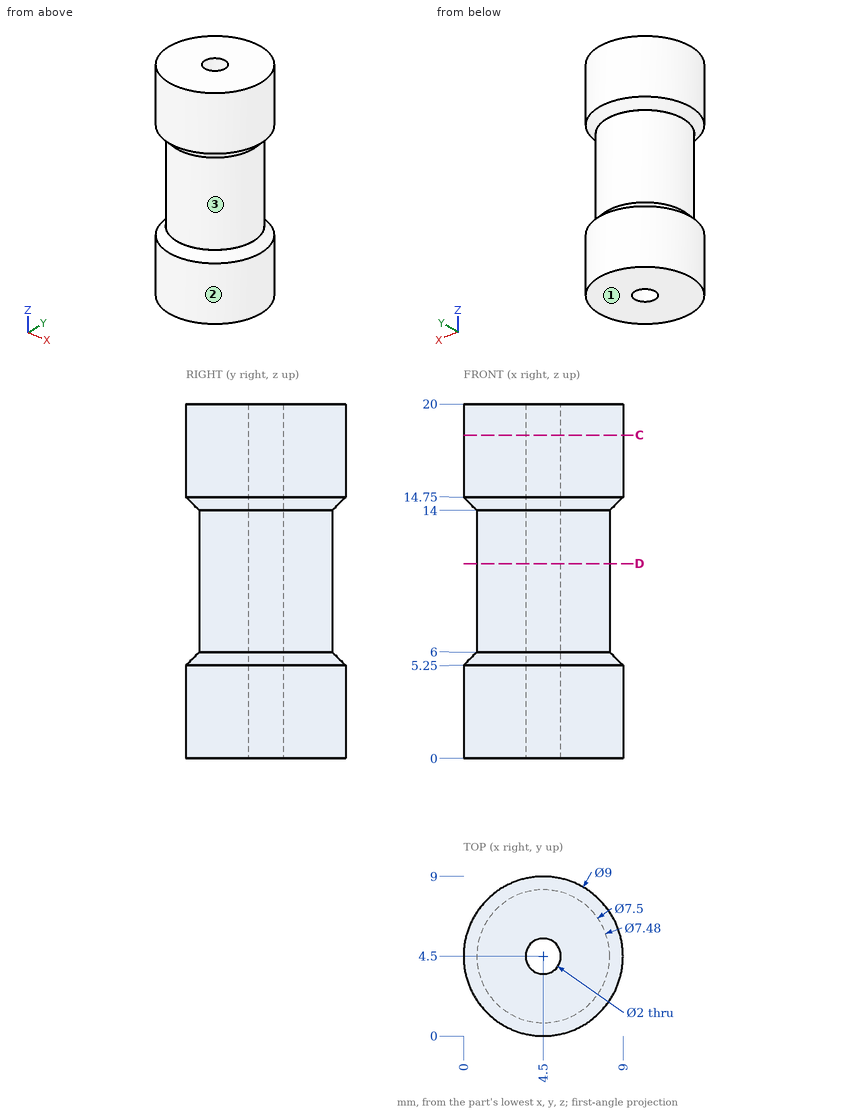
Design review of the part shown in the three views and the two pictorial views. Dimensions are in mm from the part's minimum x, y and z. Round coordinates to 2 decimals unless told otherwise and drop trailing zeros. Loops run counter-clockwise (first coordinate to the right, second up) from the corner with the lowest first, then second, coordinate; pieces in that order, holes last. Notation, with made-up numbers: (21, 42) - (29, 42) arc R28 cw to (29, 72) - close; hole circle Ø4 at (2, 74.25). An arc over 180 degrees is marked (long way). Write each question's results on one line, items separated by ' | '. Start each with the question number.
Q1. Take a section at C-C on z = 18.25. Give the boundary of the cut face in (x, y), plus the area to 3 significant figures.
Q2. Wall thickness on line 1 along Y through (x, z) = (4.5, 10); line 2 along Z through (x, y) = (1.5, 7.5); line 3 along Y through (x, z) = (4.25, 2.5): over which ranges is each line inside the solid? List them lowest first. Write a range as [from, to].
Q3. Insertion check: P1, Ø4, axis at x = 8, y = 3, coming from the -Z side; P2, Ø1.2, axis at x = 4.5, y = 4.5, coming from the -Z side; P3, Ø1.5, axis at y = 7.5, z = 4, coming from the -X side; P4, Ø1.5, axis at x = 3.5, z = 16.5, coming from the +Y side. Each pin has a flat end and moves straight along its axis. Give the tip position at first contact, or say it passes through.
Q4. Take a section at D-D on z = 11. Give the boundary of the cut face in (x, y), plus the area to 3 significant figures.
Q5. Draft analysis for pull direction Z (two halves, no side actions). For the marked faces 1, 2 and 3, state which applies: pulls with the +Z half, pulls with the -Z half, needs draft (parallel to the pull), parting line crosses it, or undercut.
Data:
1) outline: circle Ø9 at (4.5, 4.5); hole circle Ø2 at (4.5, 4.5) | area: 60.5 mm²
2) line 1: y = [0.76, 3.5], [5.5, 8.24] | line 2: z = [0, 5.51], [14.49, 20] | line 3: y = [0.01, 3.53], [5.47, 8.99]
3) P1: stops at z = 0 | P2: passes through | P3: stops at x = 0.6 | P4: stops at y = 8.99
4) outline: circle Ø7.48 at (4.5, 4.5); hole circle Ø2 at (4.5, 4.5) | area: 40.8 mm²
5) face 1: pulls with the -Z half | face 2: needs draft | face 3: undercut
